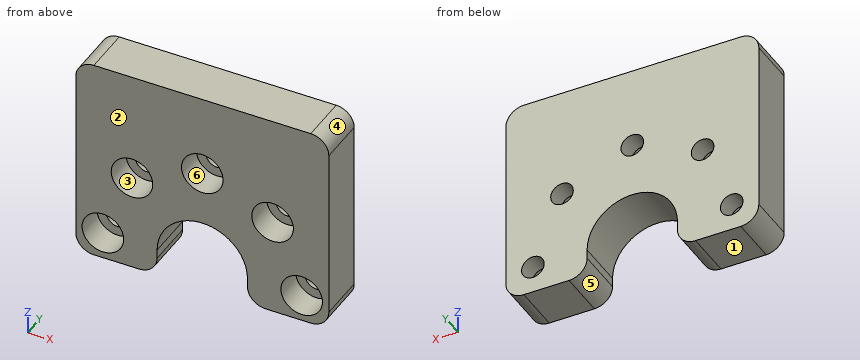
Autodesk Inventor part; units mm, degrees
ref_plane "YZ Plane" through (0, 0, 0) normal (1, 0, 0) x (0, 1, 0)
ref_plane "XZ Plane" through (0, 0, 0) normal (0, 1, 0) x (-1, 0, 0)
ref_plane "XY Plane" through (0, 0, 0) normal (0, 0, 1) x (1, 0, 0)
sketch "Sketch1" plane through (0, 0, 0) normal (0, 1, 0) x (-1, 0, 0)
  line L0 (14, 0) -> (-14, 0) construction
  line L1 (-14, 0) -> (-14, 20)
  line L2 (-14, 20) -> (14, 20)
  line L3 (14, 20) -> (14, 0)
  circle A0 centre (0, 0) radius 5
  line L4 (14, 0) -> (14, -3)
  line L5 (14, -3) -> (4, -3)
  line L6 (-14, -3) -> (-14, 0)
  line L7 (9.8995, 9.8995) -> (-9.8995, -9.8995) construction
  line L8 (0, 14) -> (0, -14) construction
  line L9 (-9.8995, 9.8995) -> (9.8995, -9.8995) construction
  line L10 (-14, 0) -> (14, 0) construction
  line L11 (-4, -3) -> (-14, -3)
  line L12 (4, -3) -> (-4, -3) construction
  line L13 (5, 0) -> (5, -1)
  line L14 (-5, 0) -> (-5, -1)
  arc A1 (-7, -3) -> (-5, -1) centre (-7, -1) ccw
  arc A2 (5, -1) -> (7, -3) centre (7, -1) ccw
  point P0 (11, 0)
  point P1 (7.7782, 7.7782)
  point P2 (0, 11)
  point P3 (-7.7782, 7.7782)
  point P4 (-11, 0)
  dimension "d0" = 28
  dimension "d1" = 10
  dimension "d2" = 20
  dimension "d3" = 3
  dimension "d4" = 11
  dimension "d7" = 180
  dimension "d20" = 1
extrude "Extrusion1" add sketch "Sketch1" along normal blind 5.3 contours L1 L2 L3 L4 L5 A2 L13 A0 L14 A1 L11 L6
hole "Hole1" at (-11, 0, 0) at (-7.7782, 0, 7.7782) at (0, 0, 11) at (7.7782, 0, 7.7782) at (11, 0, 0) direction (0, 1, 0) diameter 2.5 end through all counterbore diameter 4.6 counterbore depth 3.1
fillet "Fillet2" radius 2 4 edges at (-14, 2.65, -3) (-14, 2.65, 20) (14, 2.65, 20) (14, 2.65, -3)
equation "\"d9\" = teflon_thickness"
equation "\"d13\" = trace_radius"
equation "\"d14\" = trace_depth"
equation "\"teflon_thickness\" = 5.3"
equation "\"trace_radius\" = 4.6"
properties part number "elbow_protection"
Verification items for the finished model (mm, model axes). Face numbers are marked on the shaded views. A direction names the side the tool comes from. Coordinates: 2 decimals unless noted, no trailing zeros. Order: outer loops, then holes, each group sorted by start corner. A loop starts at its lowest first (then second) coordinate and runs counter-clockwise, first axis right, second up. Notation, with made-up numbers: (3.5, 82) -> (37.5, 82) arc R18 ccw to (37.5, 117) -> close; hole circle Ø5 at (-4.75, -19.5). An arc over 180 degrees is marked (long way). Put each result on its own line as item: value. Start each with the question number.
1. Go/stop test with a flat-tipped pin: pin 1 Ø3 at (x, z) = (0, 11) entering from -Y. Record where the tip stops, or that it passes through.
2. Cross-section at A-A, the plane x = -11. Record the boundary of the cut face in (y, z), then the cut area to 3 significant figures.
3. Cross-section at B-B, the plane z = 11. Record the boundary of the cut face in (x, y), then the cut area to 3 significant figures.
4. Mould release check, pull along Z, two halves, no side actions. Record for the marked faces 1, 2 and 3: released by +Z, released by -Z, zero draft, split by the parting line, or undercut.
5. Cross-section at D-D, the plane z = 2.75. Record the boundary of the cut face in (x, y).
6. Access from +Z, -Z, +X, -X, +Y, -Y to the whole of each face (thin tool, end or side, straight path). Record for the marked faces 4, 5 and 6.
7. Cross-section at C-C, the plane y = 0.9. Record the boundary of the cut face in (x, z).
8. Material ranges on L1, parallel to X at y = 4.7, z = 0; L2, parallel to X at y = 3.95, z = 11; L3, parallel to Z at x = -11, y = 2.8, recorded low to high. Write a range as [from, to].
Computed:
1. pin 1: y = 3.1
2. outline: (0, -3) -> (5.3, -3) -> (5.3, -1.25) -> (3.1, -1.25) -> (3.1, -2.3) -> (0, -2.3) -> close; (0, 2.3) -> (3.1, 2.3) -> (3.1, 1.25) -> (5.3, 1.25) -> (5.3, 20) -> (0, 20) -> close
2. area: 102 mm2
3. outline: (-14, 0) -> (-2.3, 0) -> (-2.3, 3.1) -> (-1.25, 3.1) -> (-1.25, 5.3) -> (-14, 5.3) -> close; (1.25, 3.1) -> (2.3, 3.1) -> (2.3, 0) -> (14, 0) -> (14, 5.3) -> (1.25, 5.3) -> close
3. area: 129 mm2
4. face 1: released by -Z
4. face 2: zero draft
4. face 3: undercut
5. outline: (-14, 0) -> (-4.18, 0) -> (-4.18, 5.3) -> (-14, 5.3) -> close; (4.18, 0) -> (14, 0) -> (14, 5.3) -> (4.18, 5.3) -> close
6. face 4: +Z, +X, +Y, -Y
6. face 5: -Z, +Y, -Y
6. face 6: -Y
7. outline: (-14, -1) arc R2 ccw to (-12, -3) -> (-7, -3) arc R2 ccw to (-5, -1) -> (-5, 0) arc R5 cw to (5, 0) -> (5, -1) arc R2 ccw to (7, -3) -> (12, -3) arc R2 ccw to (14, -1) -> (14, 18) arc R2 ccw to (12, 20) -> (-12, 20) arc R2 ccw to (-14, 18) -> close; hole circle Ø4.6 at (-11, 0); hole circle Ø4.6 at (-7.78, 7.78); hole circle Ø4.6 at (0, 11); hole circle Ø4.6 at (7.78, 7.78); hole circle Ø4.6 at (11, 0)
8. L1: [-14, -12.25], [-9.75, -5], [5, 9.75], [12.25, 14]
8. L2: [-14, -1.25], [1.25, 14]
8. L3: [-3, -2.3], [2.3, 20]
